```python
from build123d import *

# Parameters (mm, degrees)
SKETCH1_R            = 21.082
SKETCH1_R_2          = 17.526
BOSS_EXTRUDE1_DEPTH  = 254
BOSS_EXTRUDE2_START  = 6.35
SKETCH2_R            = 21.082
BOSS_EXTRUDE2_DEPTH  = 6.35
SKETCH3_R            = 25.868376463
CUT_EXTRUDE1_DEPTH   = 127
SKETCH4_R            = 34.925
SKETCH4_R_2          = 19.091061219
BOSS_EXTRUDE3_DEPTH  = 3.175
CUT_EXTRUDE2_DEPTH   = 143.203142546
CIRPATTERN1_COUNT    = 12
SKETCH6_R            = 21.082
CUT_EXTRUDE3_DEPTH   = 6.35
SKETCH7_R            = 21.082
BOSS_EXTRUDE4_DEPTH  = 6.35
CUT_EXTRUDE5_DEPTH   = 137.26632471
BOSS_EXTRUDE5_DEPTH  = 3.175
SKETCH13_R           = 20.701
SKETCH13_R_2         = 18.0848
CUT_EXTRUDE6_DEPTH   = 1.016
SKETCH14_R           = 22.3012
SKETCH14_R_2         = 20.701
BOSS_EXTRUDE6_DEPTH  = 3.175
SKETCH15_R           = 3.175
SKETCH15_R_2         = 21.082
BOSS_EXTRUDE7_DEPTH  = 123.825
SKETCH17_R           = 47.464750001
SKETCH17_R_2         = 22.3012
CUT_EXTRUDE7_DEPTH   = 120.65
SKETCH18_R           = 17.526
CUT_EXTRUDE8_DEPTH   = 134.883658048
CUT_EXTRUDE9_START   = -1.016
SKETCH19_R           = 20.701
SKETCH19_R_2         = 18.0848
CUT_EXTRUDE9_DEPTH   = 1.016
SKETCH20_R           = 44.795310745
SKETCH20_R_2         = 22.3012
CUT_EXTRUDE10_DEPTH  = 12.7
BOSS_EXTRUDE8_START  = 31.75
SKETCH22_R           = 22.3012
SKETCH22_R_2         = 20.701
SKETCH22_R_3         = 18.0848
SKETCH22_R_4         = 17.526
BOSS_EXTRUDE8_DEPTH  = 31.75
BOSS_EXTRUDE9_START  = 32.766
SKETCH23_R           = 20.701
SKETCH23_R_2         = 18.0848
BOSS_EXTRUDE9_DEPTH  = 32.766
SKETCH24_R           = 17.526
BOSS_EXTRUDE10_DEPTH = 6.35
SKETCH25_R           = 3.2385
CUT_EXTRUDE11_DEPTH  = 165.308844535


with BuildPart() as part:
    # Sketch1 → Boss-Extrude1 (new body)
    with BuildSketch(Plane.XY):
        Circle(SKETCH1_R)
        Circle(SKETCH1_R_2, mode=Mode.SUBTRACT)
    extrude(amount=BOSS_EXTRUDE1_DEPTH)

    # Sketch2 → Boss-Extrude2 (add)
    with BuildSketch(Plane(origin=(0, 0, 0), x_dir=(-1, 0, 0), z_dir=(0, 0, -1)).offset(BOSS_EXTRUDE2_START)):
        Circle(SKETCH2_R)
    extrude(amount=-BOSS_EXTRUDE2_DEPTH)

    # Sketch3 → Cut-Extrude1 (cut)
    with BuildSketch(Plane.XY.offset(254)):
        Circle(SKETCH3_R)
    extrude(amount=-CUT_EXTRUDE1_DEPTH, mode=Mode.SUBTRACT)

    # Sketch4 → Boss-Extrude3 (add)
    with BuildSketch(Plane.XY.offset(127)):
        Circle(SKETCH4_R)
        Circle(SKETCH4_R_2, mode=Mode.SUBTRACT)
    extrude(amount=-BOSS_EXTRUDE3_DEPTH)

    # Sketch5 → Cut-Extrude2 (cut, through all)
    with BuildSketch(Plane.XY.offset(127)):
        with BuildLine():
            ThreePointArc((0, 31.75), (-3.175, 28.575), (0, 25.4))
            Line((0, 25.4), (0, 31.75))
        make_face()
        with BuildLine():
            Line((0, 31.75), (0, 25.4))
            ThreePointArc((0, 25.4), (2.24506403, 26.32993597), (3.175, 28.575))
            ThreePointArc((3.175, 28.575), (2.24506403, 30.82006403), (0, 31.75))
        make_face()
    cut_extrude2 = extrude(amount=-CUT_EXTRUDE2_DEPTH, mode=Mode.SUBTRACT)

    # CirPattern1: Cut-Extrude2 ×12 about axis
    cirpattern1_axis = Axis((0, 0, 0), (0, 0, 1))
    for i in range(1, CIRPATTERN1_COUNT):
        add(cut_extrude2.rotate(cirpattern1_axis, i * 360 / CIRPATTERN1_COUNT), mode=Mode.SUBTRACT)

    # Sketch6 → Cut-Extrude3 (cut)
    with BuildSketch(Plane(origin=(0, 0, -6.35), x_dir=(-1, 0, 0), z_dir=(0, 0, -1))):
        Circle(SKETCH6_R)
    extrude(amount=-CUT_EXTRUDE3_DEPTH, mode=Mode.SUBTRACT)

    # Sketch7 → Boss-Extrude4 (add)
    with BuildSketch(Plane(origin=(0, 0, 0), x_dir=(-1, 0, 0), z_dir=(0, 0, -1))):
        Circle(SKETCH7_R)
    extrude(amount=-BOSS_EXTRUDE4_DEPTH)

    # Sketch8 → Cut-Extrude5 (cut, through all)
    with BuildSketch(Plane.XY.offset(127)):
        with BuildLine():
            ThreePointArc((18.828599641, 18.828599641), (22.949516837, 21.527350272), (27.854121372, 21.069018667))
            ThreePointArc((27.854121372, 21.069018667), (0, 34.925), (-27.854121372, 21.069018667))
            ThreePointArc((-27.854121372, 21.069018667), (-22.949516837, 21.527350272), (-18.828599641, 18.828599641))
            Line((-18.828599641, 18.828599641), (-14.907225161, 14.907225161))
            ThreePointArc((-14.907225161, 14.907225161), (0, 21.082), (14.907225161, 14.907225161))
            Line((14.907225161, 14.907225161), (18.828599641, 18.828599641))
        make_face()
        with BuildLine():
            ThreePointArc((14.907225161, -14.907225161), (0, -21.082), (-14.907225161, -14.907225161))
            Line((-14.907225161, -14.907225161), (-18.828599641, -18.828599641))
            ThreePointArc((-18.828599641, -18.828599641), (-22.949516837, -21.527350272), (-27.854121372, -21.069018667))
            ThreePointArc((-27.854121372, -21.069018667), (0, -34.925), (27.854121372, -21.069018667))
            ThreePointArc((27.854121372, -21.069018667), (22.949516837, -21.527350272), (18.828599641, -18.828599641))
            Line((18.828599641, -18.828599641), (14.907225161, -14.907225161))
        make_face()
    extrude(amount=-CUT_EXTRUDE5_DEPTH, mode=Mode.SUBTRACT)

    # Sketch11 → Boss-Extrude5 (add)
    with BuildSketch(Plane.XY.offset(127)):
        with BuildLine():
            ThreePointArc((31.206854634, 18.017286001), (29.767943301, 19.804028486), (27.854121372, 21.069018667))
            ThreePointArc((27.854121372, 21.069018667), (34.925, 0), (27.854121372, -21.069018667))
            ThreePointArc((27.854121372, -21.069018667), (29.767943301, -19.804028486), (31.206854634, -18.017286001))
            ThreePointArc((31.206854634, -18.017286001), (36.034571885, 0), (31.206854634, 18.017286001))
        make_face()
        with BuildLine():
            ThreePointArc((-27.854121372, 21.069018667), (-29.767943301, 19.804028486), (-31.206854634, 18.017286001))
            ThreePointArc((-31.206854634, 18.017286001), (-36.034571885, -1.77e-07), (-31.206854456, -18.017286308))
            ThreePointArc((-31.206854456, -18.017286308), (-29.767943169, -19.804028605), (-27.854121372, -21.069018667))
            ThreePointArc((-27.854121372, -21.069018667), (-34.925, 0), (-27.854121372, 21.069018667))
        make_face()
    extrude(amount=-BOSS_EXTRUDE5_DEPTH)

    # Sketch13 → Cut-Extrude6 (cut)
    with BuildSketch(Plane.XY.offset(127)):
        Circle(SKETCH13_R)
        Circle(SKETCH13_R_2, mode=Mode.SUBTRACT)
    extrude(amount=-CUT_EXTRUDE6_DEPTH, mode=Mode.SUBTRACT)

    # Sketch14 → Boss-Extrude6 (add)
    with BuildSketch(Plane.XY.offset(127)):
        Circle(SKETCH14_R)
        Circle(SKETCH14_R_2, mode=Mode.SUBTRACT)
    extrude(amount=-BOSS_EXTRUDE6_DEPTH)

    # Sketch15 → Boss-Extrude7 (add)
    with BuildSketch(Plane(origin=(0, 0, 123.825), x_dir=(-1, 0, 0), z_dir=(0, 0, -1))):
        with BuildLine():
            ThreePointArc((31.206854667, 18.017285943), (25.234555257, 21.731100369), (18.828599641, 18.828599641))
            Line((18.828599641, 18.828599641), (15.769329749, 15.769329749))
            ThreePointArc((15.769329749, 15.769329749), (0, 22.3012), (-15.769329749, 15.769329749))
            Line((-15.769329749, 15.769329749), (-18.828599641, 18.828599641))
            ThreePointArc((-18.828599641, 18.828599641), (-25.234555257, 21.731100369), (-31.206854667, 18.017285943))
            ThreePointArc((-31.206854667, 18.017285943), (-36.034571885, 0), (-31.206854667, -18.017285943))
            ThreePointArc((-31.206854667, -18.017285943), (-25.234555257, -21.731100369), (-18.828599641, -18.828599641))
            Line((-18.828599641, -18.828599641), (-15.769329749, -15.769329749))
            ThreePointArc((-15.769329749, -15.769329749), (0, -22.3012), (15.769329749, -15.769329749))
            Line((15.769329749, -15.769329749), (18.828599641, -18.828599641))
            ThreePointArc((18.828599641, -18.828599641), (25.234555257, -21.731100369), (31.206854667, -18.017285943))
            ThreePointArc((31.206854667, -18.017285943), (36.034571885, 0), (31.206854667, 18.017285943))
        make_face()
        with Locations(Location((28.575, 0, 0), (0, 0, 90))):
            Circle(SKETCH15_R, mode=Mode.SUBTRACT)
        with Locations(Location((-24.746675913, -14.2875, 0), (0, 0, 300))):
            Circle(SKETCH15_R, mode=Mode.SUBTRACT)
        with Locations(Location((-24.746675913, 14.2875, 0), (0, 0, 240))):
            Circle(SKETCH15_R, mode=Mode.SUBTRACT)
        with Locations(Location((-28.575, 0, 0), (0, 0, 270))):
            Circle(SKETCH15_R, mode=Mode.SUBTRACT)
        Circle(SKETCH15_R_2, mode=Mode.SUBTRACT)
        with Locations(Location((24.746675913, -14.2875, 0), (0, 0, 60))):
            Circle(SKETCH15_R, mode=Mode.SUBTRACT)
        with Locations(Location((24.746675913, 14.2875, 0), (0, 0, 120))):
            Circle(SKETCH15_R, mode=Mode.SUBTRACT)
    extrude(amount=BOSS_EXTRUDE7_DEPTH)

    # Sketch17 → Cut-Extrude7 (cut)
    with BuildSketch(Plane.XY.offset(123.825)):
        Circle(SKETCH17_R)
        with Locations(Location((0, 0, 0), (0, 0, 315))):
            Circle(SKETCH17_R_2, mode=Mode.SUBTRACT)
    extrude(amount=-CUT_EXTRUDE7_DEPTH, mode=Mode.SUBTRACT)

    # Sketch18 → Cut-Extrude8 (cut, through all)
    with BuildSketch(Plane.XY.offset(127)):
        Circle(SKETCH18_R)
    extrude(amount=-CUT_EXTRUDE8_DEPTH, mode=Mode.SUBTRACT)

    # Sketch19 → Cut-Extrude9 (cut)
    with BuildSketch(Plane(origin=(0, 0, 0), x_dir=(-1, 0, 0), z_dir=(0, 0, -1)).offset(CUT_EXTRUDE9_START)):
        with Locations(Location((0, 0, 0), (0, 0, 180))):
            Circle(SKETCH19_R)
        with Locations(Location((0, 0, 0), (0, 0, 180))):
            Circle(SKETCH19_R_2, mode=Mode.SUBTRACT)
    extrude(amount=CUT_EXTRUDE9_DEPTH, mode=Mode.SUBTRACT)

    # Sketch20 → Cut-Extrude10 (cut)
    with BuildSketch(Plane.XY.offset(127)):
        Circle(SKETCH20_R)
        Circle(SKETCH20_R_2, mode=Mode.SUBTRACT)
    extrude(amount=-CUT_EXTRUDE10_DEPTH, mode=Mode.SUBTRACT)

    # Sketch22 → Boss-Extrude8 (add)
    # profile 1 of 2: a face of its own
    with BuildSketch(Plane.XY.offset(127).offset(BOSS_EXTRUDE8_START)):
        Circle(SKETCH22_R)
        Circle(SKETCH22_R_2, mode=Mode.SUBTRACT)
    # profile 2 of 2: a face of its own
    with BuildSketch(Plane.XY.offset(127).offset(BOSS_EXTRUDE8_START)):
        Circle(SKETCH22_R_3)
        Circle(SKETCH22_R_4, mode=Mode.SUBTRACT)
    extrude(amount=-BOSS_EXTRUDE8_DEPTH)

    # Sketch23 → Boss-Extrude9 (add)
    with BuildSketch(Plane.XY.offset(125.984).offset(BOSS_EXTRUDE9_START)):
        with Locations(Location((0, 0, 0), (0, 0, 180))):
            Circle(SKETCH23_R)
        with Locations(Location((0, 0, 0), (0, 0, 180))):
            Circle(SKETCH23_R_2, mode=Mode.SUBTRACT)
    extrude(amount=-BOSS_EXTRUDE9_DEPTH)

    # Sketch24 → Boss-Extrude10 (add)
    with BuildSketch(Plane.XY.offset(158.75)):
        Circle(SKETCH24_R)
    extrude(amount=-BOSS_EXTRUDE10_DEPTH)

    # Sketch25 → Cut-Extrude11 (cut, through all)
    with BuildSketch(Plane(origin=(0, 0, 0), x_dir=(-1, 0, 0), z_dir=(0, 0, -1))):
        with Locations((-24.746675913, 14.2875)):
            Circle(SKETCH25_R)
        with Locations((-28.575, 0)):
            Circle(SKETCH25_R)
        with Locations((-24.746675913, -14.2875)):
            Circle(SKETCH25_R)
        with Locations((24.746675913, 14.2875)):
            Circle(SKETCH25_R)
        with Locations((28.575, 0)):
            Circle(SKETCH25_R)
        with Locations((24.746675913, -14.2875)):
            Circle(SKETCH25_R)
    extrude(amount=-CUT_EXTRUDE11_DEPTH, mode=Mode.SUBTRACT)


solid = part.part
```
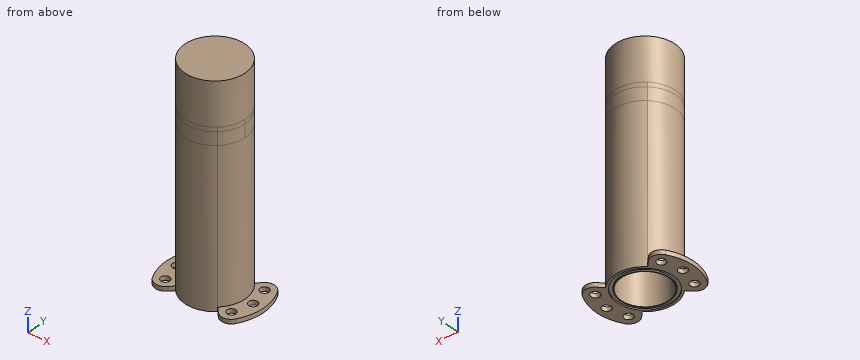
The model under review builds one solid part; all positions refer to its coordinate system, in mm. Coordinates: 2 decimals unless noted, no trailing zeros. Write each loop counter-clockwise with the first axis right and the second up, starting at its lowest first coordinate (ties: lowest second). Pieces come first, ordered by that corner, then holes.
1) To check wall thickness, follow probe 1 along Z at (x, y) = (-20.5, -2); probe 2 along X at (y, z) = (7, 78.5); probe 3 along Y at (x, z) = (-1, 94.5). State the ranges of each line that lie inside material, in increasing order.
2) We need section C-C on y = -7.5. State the section outline as (x, z) points (3 decimals), then the cut area to 3 significant figures.
3) We need section B-B on z = 43.5. State the section outline as (x, y) points, then the cut area to 3 significant figures.
4) We need section A-A on x = 0. State the section outline as (y, z) points, then the cut area to 3 significant figures.
5) Clearance check with flat-ended pins moving along their axes: pin 1 Ø1.5 at (x, y) = (-6.5, -15) entering from -Z; pin 2 Ø10.5 at (x, y) = (24.75, 14.29) entering from +Z (3 decimals); pin 3 Ø10 at (x, z) = (9.5, 112) entering from -Y. State where each tip first meets the part, or that it passes through.
6) We need section D-D on x = -8. State the section outline as (y, z) points (3 decimals).
Answer list:
1. probe 1: z = 1.02 to 158.75
1. probe 2: x = -21.17 to -16.07, 16.07 to 21.17
1. probe 3: y = -22.28 to -17.5, 17.5 to 22.28
2. outline: (-35.245, 0) - (-19.295, 0) - (-19.295, 1.016) - (-16.456, 1.016) - (-16.456, 0) - (-15.84, 0) - (-15.84, 152.4) - (15.84, 152.4) - (15.84, 0) - (16.456, 0) - (16.456, 1.016) - (19.295, 1.016) - (19.295, 0) - (35.245, 0) - (35.245, 3.175) - (21.002, 3.175) - (21.002, 158.75) - (-21.002, 158.75) - (-21.002, 3.175) - (-35.245, 3.175) - close
2. area: 1,920 mm2
3. outline: circle Ø44.6 at (0, 0); hole circle Ø35.05 at (0, 0)
3. area: 597 mm2
4. outline: (-22.3, 0) - (-20.7, 0) - (-20.7, 1.02) - (-18.08, 1.02) - (-18.08, 0) - (-17.53, 0) - (-17.53, 152.4) - (17.53, 152.4) - (17.53, 0) - (18.08, 0) - (18.08, 1.02) - (20.7, 1.02) - (20.7, 0) - (22.3, 0) - (22.3, 158.75) - (-22.3, 158.75) - close
4. area: 1,730 mm2
5. pin 1: stops at z = 152.4
5. pin 2: stops at z = 3.175
5. pin 3: stops at y = -21.84
6. outline: (-20.817, 0) - (-19.093, 0) - (-19.093, 1.016) - (-16.219, 1.016) - (-16.219, 0) - (-15.594, 0) - (-15.594, 152.4) - (15.594, 152.4) - (15.594, 0) - (16.219, 0) - (16.219, 1.016) - (19.093, 1.016) - (19.093, 0) - (20.817, 0) - (20.817, 158.75) - (-20.817, 158.75) - close
